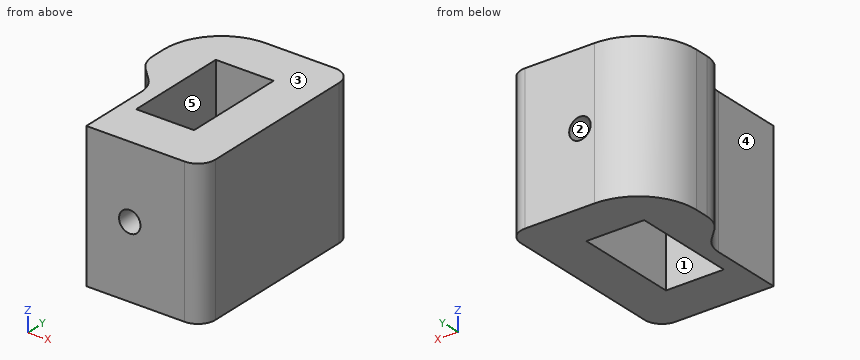
```python
from build123d import *

# Parameters (mm, degrees)
F0_W     = 10
F0_H     = 18
F1_DEPTH = 25
F2_R     = 5
F3_R     = 1.85
F4_DEPTH = 50
F5_R     = 10
F6_R     = 3


with BuildPart() as f1:
    # F0 (on Top) → F1 (new body)
    with BuildSketch(Plane.XY):
        Polygon((-7.5, 0), (0, 0), (7.5, 0), (12.5, 0), (12.5, 19.5), (12.5, 34), (0, 34), (-12.5, 34), (-12.5, 19.5), (-7.5, 14.5), align=None)
        with Locations((0, 17)):
            Rectangle(F0_W, F0_H, mode=Mode.SUBTRACT)
    extrude(amount=F1_DEPTH)

    # F2
    f2_edges = [f1.edges().sort_by_distance(p)[0] for p in [
        (-12.5, 19.5, 12.5),
        (-7.5, 14.5, 12.5),
    ]]
    fillet(f2_edges, radius=F2_R)

    # F3 (on face) → F4 (cut, symmetric)
    with BuildSketch(Plane(origin=(0, 8, 0), x_dir=(-1, 0, 0), z_dir=(0, 1, 0))):
        with Locations((0, 12.5)):
            Circle(F3_R)
    extrude(amount=F4_DEPTH, both=True, mode=Mode.SUBTRACT)

    # F5
    f5_edges = [f1.edges().sort_by_distance(p)[0] for p in [
        (-12.5, 34, 12.5),
    ]]
    fillet(f5_edges, radius=F5_R)

    # F6
    f6_edges = [f1.edges().sort_by_distance(p)[0] for p in [
        (12.5, 34, 12.5),
        (12.5, 0, 12.5),
    ]]
    fillet(f6_edges, radius=F6_R)


solid = f1.part
```
Work out the finished part from the listing and answer in its coordinate system (mm). Face numbers are marked on the shaded views. A direction names the side the tool comes from. Coordinates: 2 decimals unless noted, no trailing zeros. Loops run counter-clockwise (first coordinate to the right, second up) from the corner with the lowest first, then second, coordinate; pieces in that order, holes last.
1) Flat-ended cylindrical pins translate along their axes: pin 1 (8 mm diameter, centred on x = -3, y = 23.5, fed in from -Z); pin 2 (5.5 mm diameter, centred on y = 16.5, z = 8.5, fed in from -X); pin 3 (6 mm diameter, centred on y = 7.5, z = 13.5, fed in from -X). Find the tip coordinate at first contact, or state that the pin passes through.
Results:
pin 1: stops at z = 0
pin 2: stops at x = -11.93
pin 3: stops at x = -7.5
2) Consider probe 1 along Z at (x, y) = (0, 2.25); probe 2 along X at (y, z) = (10.5, 3.75); probe 3 along Y at (x, z) = (2.5, 22.75). Determine where each line is inside the solid, lowest interval first.
Results:
probe 1: z = 0 to 10.65, 14.35 to 25
probe 2: x = -7.5 to -5, 5 to 12.5
probe 3: y = 0 to 8, 26 to 34
3) For the marked faces 1 and 2, determine the directions among +Z, -Z, +X, -X, +Y, -Y from which every point of the face is accessible in a straight line to the end or side of a thin tool.
Results:
face 1: +Z, -Z
face 2: +Y, -Y
4) Section C-C (y = 25) is taken. Give the vertices of the cut face in (x, z).
Results:
outline: (-12.45, 0) - (-5, 0) - (-5, 25) - (-12.45, 25) - close; (5, 0) - (12.5, 0) - (12.5, 25) - (5, 25) - close
5) Section A-A (x = 0) is taken. Give the vertices of the cut face in (y, z), plus the area to 3 significant figures.
Results:
outline: (0, 0) - (8, 0) - (8, 10.65) - (0, 10.65) - close; (0, 14.35) - (8, 14.35) - (8, 25) - (0, 25) - close; (26, 0) - (34, 0) - (34, 10.65) - (26, 10.65) - close; (26, 14.35) - (34, 14.35) - (34, 25) - (26, 25) - close
area: 341 mm2
6) Section D-D (z = 12.5) is taken. Give the vertices of the cut face in (x, y).
Results:
outline: (-12.5, 21.57) arc R5 ccw to (-11.04, 18.04) - (-8.96, 15.96) arc R5 cw to (-7.5, 12.43) - (-7.5, 0) - (-1.85, 0) - (-1.85, 8) - (-5, 8) - (-5, 26) - (-1.85, 26) - (-1.85, 34) - (-2.5, 34) arc R10 ccw to (-12.5, 24) - close; (1.85, 0) - (9.5, 0) arc R3 ccw to (12.5, 3) - (12.5, 31) arc R3 ccw to (9.5, 34) - (1.85, 34) - (1.85, 26) - (5, 26) - (5, 8) - (1.85, 8) - close
7) For a pull along X with two mould halves and no side action, classify the marked faces 3, 4 and 5 as +X half, -X half, draft (parallel to the pull), parting line (faces both ways), or undercut.
Results:
face 3: draft
face 4: -X half
face 5: undercut
8) Section B-B (z = 2.75) is taken. Give the vertices of the cut face in (x, y).
Results:
outline: (-12.5, 21.57) arc R5 ccw to (-11.04, 18.04) - (-8.96, 15.96) arc R5 cw to (-7.5, 12.43) - (-7.5, 0) - (9.5, 0) arc R3 ccw to (12.5, 3) - (12.5, 31) arc R3 ccw to (9.5, 34) - (-2.5, 34) arc R10 ccw to (-12.5, 24) - close; hole (-5, 8) - (5, 8) - (5, 26) - (-5, 26) - close
